Source: CAD feature listing. Evaluate the final solid. Frame: model axes, mm. A direction names the side the tool comes from. Give positions to 0.01 mm unless a question says otherwise; leave off trailing zeros. Loops run counter-clockwise (first coordinate to the right, second up) from the corner with the lowest first, then second, coordinate; pieces in that order, holes last. Notation, with made-up numbers: (34.25, 56) -> (43.25, 56) arc R28 ccw to (43.25, 87) -> close; hole circle Ø2 at (-38, 63). An arc over 180 degrees is marked (long way). Return JSON: item names as keys, results as strings. Group by question number.
(1) Pin query (flat end, axial travel): pin 1 (2 mm diameter, centred on y = 17, z = -2, fed in from +X); pin 2 (1.5 mm diameter, centred on y = -10.5, z = 0, fed in from -X). Return the tip coordinate at first contact, or that it passes through.
(2) Cut plane B-B on y = 14. Return loops of the section in (x, z) (3 decimals), then the cut area to 3 significant figures.
(3) Ray query, line 1 (X direction, y = 7.5, z = 0); line 2 (X direction, y = -6.5, z = -2.5); line 3 (X direction, y = 22, z = 1). Return the intervals inside material, ascending. Write a range as from..to.
(4) Cut plane C-C on x = 3.5. Return loops of the section in (y, z) (3 decimals).
(5) Cut plane A-A on z = 1.75. Return loops of the section in (x, y), then the cut area to 3 significant figures.
(6) Cut plane D-D on y = 2.5. Return loops of the section in (x, z) (3 decimals).
(7) Draft query along X for faces 1 (the face through (14.85, 4.15, 0.04)), 2 (the face through (19, -21.609, 0)), 3 (the face through (0, 5.704, 0)). Return one class per face: released by +X, released by -X, zero draft, split by the parting line, or undercut.
(8) Access query for faces 4 (the face through (10.201, -10.956, 0.044)), 5 (the face through (-2.47, 12.21, 0.04)), 6 (the face through (1, 4, 3.175)). Directions: +Z, -Z, +X, -X, +Y, -Y. A direction counts if a zero-diameter tool reaches every point of the face in a straight line with its end or side. Return the directions, or none.
```python
from build123d import *

# Parameters (mm, degrees)
BOSS_EXTRUDE1_DEPTH = 3.175


with BuildPart() as part:
    # Sketch1 → Boss-Extrude1 (new body, symmetric)
    with BuildSketch(Plane.XY):
        Polygon((-5.278441348, 29.190879636), (5.278441348, 29.190879636), (24.698908797, -21.609120364), (13.966676058, -21.609120364), (6.328370689, 0), (-6.328370689, 0), (-13.154027538, -21.609120364), (-23.886260277, -21.609120364), align=None)
        Polygon((-0.355555483, 18.909137327), (4.312269234, 5.703644579), (-4.526764699, 5.703644579), align=None, mode=Mode.SUBTRACT)
    extrude(amount=BOSS_EXTRUDE1_DEPTH, both=True)


solid = part.part
```
Answers:
{
 "1": {"pin 1": "x = 10.32", "pin 2": "x = -20.09"},
 "2": {"outline": "(-10.843, -3.175) -> (-1.906, -3.175) -> (-1.906, 3.175) -> (-10.843, 3.175) -> close; (1.38, -3.175) -> (11.086, -3.175) -> (11.086, 3.175) -> (1.38, 3.175) -> close", "area": "118 mm²"},
 "3": {"line 1": "-13.22..-3.96, 3.68..13.57", "line 2": "-18.35..-8.38, 8.63..18.92", "line 3": "-7.91..8.03"},
 "4": {"outline": "(0, -3.175) -> (5.704, -3.175) -> (5.704, 3.175) -> (0, 3.175) -> close; (8.002, -3.175) -> (29.191, -3.175) -> (29.191, 3.175) -> (8.002, 3.175) -> close"},
 "5": {"outline": "(-23.89, -21.61) -> (-13.15, -21.61) -> (-6.33, 0) -> (6.33, 0) -> (13.97, -21.61) -> (24.7, -21.61) -> (5.28, 29.19) -> (-5.28, 29.19) -> close; hole (-4.53, 5.7) -> (4.31, 5.7) -> (-0.36, 18.91) -> close", "area": "1,010 mm²"},
 "6": {"outline": "(-15.055, -3.175) -> (15.482, -3.175) -> (15.482, 3.175) -> (-15.055, 3.175) -> close"},
 "7": {"face 1": "released by +X", "face 2": "zero draft", "face 3": "undercut"},
 "8": {"face 4": "+Z, -Z, -Y", "face 5": "+Z, -Z", "face 6": "+Z, +X, -X, +Y, -Y"}
}
